Part model, mm, in its own coordinate system. Round coordinates to 2 decimals unless told otherwise and drop trailing zeros. Loops run counter-clockwise (first coordinate to the right, second up) from the corner with the lowest first, then second, coordinate; pieces in that order, holes last.
(1) Cut at D-D on z = 51.5. List the corners of the cut face in (x, y).
(2) Flat gauge pins, fed straight in: pin 1 (16.5 mm diameter, centred on x = -44.45, y = 19.05, fed in from +Z); pin 2 (3 mm diameter, centred on x = 3, z = 53, fed in from +Y). Where does each tip first touch, or does it go through?
(3) Probe probe 1 along X at (y, z) = (19, 6); probe 2 along Y at (x, z) = (44.45, 7); probe 3 along Z at (x, y) = (37.5, 18). List the from-to ranges inside material, lowest first.
(4) Cut at C-C on x = 55.5. List the corners of the cut face in (y, z), then the cut area to 3 significant figures.
(5) Mould opens along X. For faces 1 (the face through (63.5, -1, 10)), 2 (the face through (-38.584, -21.482, 12.878)), 3 (the face through (-1, -38.1, 10)) say: +X half, -X half, draft (parallel to the pull), parting line (faces both ways), or undercut.
(6) Cut at B-B on x = -44.45. List the corners of the cut face in (y, z), then the cut area to 3 significant figures.
from build123d import *

# Parameters (mm, degrees)
F1_DEPTH = 25.4
F2_R     = 6.35
F3_DEPTH = 25.4
F4_W     = 25.4
F4_H     = 12.7
F6_W     = 19.05
F6_H     = 19.05
F8_W     = 25.4
F8_H     = 12.7
F11_R    = 6.34999
F12_SIZE = 5.08


# Not quite as in the source:
# - a fillet or chamfer is up to 0.001 mm smaller than in the source, because OpenCascade refuses the exact size
# - a feature of the source that left no trace in its solid (it failed there, or was rolled back) is left out


with BuildPart() as f1:
    # F0 (on Top) → F1 (new body)
    with BuildSketch(Plane.XY):
        Polygon((-63.0538856602, 38.1), (-63.5, 38.1), (-63.5, -38.1), (63.5, -38.1), (63.5, 38.1), align=None)
    extrude(amount=F1_DEPTH)

    # F2 (on face) → F3 (cut)
    with BuildSketch(Plane.XY.offset(25.4)):
        with Locations((-44.45, 19.05)):
            Circle(F2_R)
        with Locations((-44.45, -19.05)):
            Circle(F2_R)
        with Locations((44.45, 19.05)):
            Circle(F2_R)
        with Locations((44.45, -19.05)):
            Circle(F2_R)
    extrude(amount=-F3_DEPTH, mode=Mode.SUBTRACT)

    # F4 (on Front) → F5 (revolve)
    with BuildSketch(Plane.XZ):
        with Locations((12.7, 31.75)):
            Rectangle(F4_W, F4_H)
    revolve(axis=Axis((0, 0, 31.75), (0, 0, -1)))

    # F6 (on Front) → F7 (revolve)
    with BuildSketch(Plane.XZ):
        with Locations((9.525, 47.625)):
            Rectangle(F6_W, F6_H)
    revolve(axis=Axis((0, 0, 47.625), (0, 0, 1)))

    # F8 (on Front) → F9 (revolve)
    with BuildSketch(Plane.XZ):
        with Locations((12.7, 63.5)):
            Rectangle(F8_W, F8_H)
    revolve(axis=Axis((0, 0, 63.5), (0, 0, 1)))

    # F11 (radius 6.35 in the source; OpenCascade refuses exactly that, so slightly less here)
    f11_edges = [f1.edges().sort_by_distance(p)[0] for p in [
        (-25.4, 0, 69.85),
        (-25.4, 0, 38.1),
        (-25.4, 0, 57.15),
        (-25.4, 0, 25.4),
        (25.4, 0, 31.75),
    ]]
    fillet(f11_edges, radius=F11_R)

    # F12
    f12_edges = [f1.edges().sort_by_distance(p)[0] for p in [
        (-63.5, 0, 25.4),
        (0, 38.1, 25.4),
        (0, -38.1, 25.4),
        (63.5, 0, 25.4),
    ]]
    chamfer(f12_edges, length=F12_SIZE)


solid = f1.part
Final values:
1. outline: circle Ø38.1 at (0, 0)
2. pin 1: stops at z = 25.4
2. pin 2: stops at y = 18.99
3. probe 1: x = -63.5 to -50.8, -38.1 to 38.1, 50.8 to 63.5
3. probe 2: y = -38.1 to -25.4, -12.7 to 12.7, 25.4 to 38.1
3. probe 3: z = 0 to 25.4
4. outline: (-38.1, 0) - (38.1, 0) - (38.1, 20.32) - (33.02, 25.4) - (-33.02, 25.4) - (-38.1, 20.32) - close
4. area: 1,910 mm2
5. face 1: +X half
5. face 2: undercut
5. face 3: draft
6. outline: (-38.1, 0) - (-25.4, 0) - (-25.4, 25.4) - (-33.02, 25.4) - (-38.1, 20.32) - close; (-12.7, 0) - (12.7, 0) - (12.7, 25.4) - (-12.7, 25.4) - close; (25.4, 0) - (38.1, 0) - (38.1, 20.32) - (33.02, 25.4) - (25.4, 25.4) - close
6. area: 1,260 mm2
